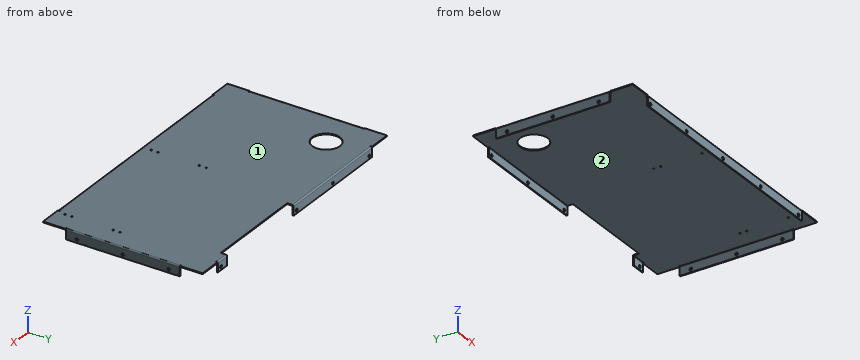
```python
from build123d import *

# Parameters (mm, degrees)
SM_BASE_FLANGE_1_DEPTH            = 2
SM_EDGE_FLANGE_1_STRIP_W          = 9.4732
SM_EDGE_FLANGE_1_STRIP_H          = 2
SM_EDGE_FLANGE_1_STRIP_CUT_DEPTH  = 248
SM_EDGE_FLANGE_1_RELIEF_W         = 10.4732
SM_EDGE_FLANGE_1_RELIEF_H         = 1
SM_EDGE_FLANGE_1_RELIEF_CUT_DEPTH = 2
SM_EDGE_FLANGE_1_DEPTH            = 248
SM_EDGE_FLANGE_2_STRIP_W          = 9.4732
SM_EDGE_FLANGE_2_STRIP_H          = 2
SM_EDGE_FLANGE_2_STRIP_CUT_DEPTH  = 510
SM_EDGE_FLANGE_2_RELIEF_W         = 10.4732
SM_EDGE_FLANGE_2_RELIEF_H         = 1
SM_EDGE_FLANGE_2_RELIEF_CUT_DEPTH = 2
SM_EDGE_FLANGE_2_DEPTH            = 510
SM_EDGE_FLANGE_3_STRIP_W          = 9.4732
SM_EDGE_FLANGE_3_STRIP_H          = 2
SM_EDGE_FLANGE_3_STRIP_CUT_DEPTH  = 248
SM_EDGE_FLANGE_3_RELIEF_W         = 10.4732
SM_EDGE_FLANGE_3_RELIEF_H         = 1
SM_EDGE_FLANGE_3_RELIEF_CUT_DEPTH = 2
SM_EDGE_FLANGE_3_DEPTH            = 248
SM_EDGE_FLANGE_4_STRIP_W          = 9.4732
SM_EDGE_FLANGE_4_STRIP_H          = 2
SM_EDGE_FLANGE_4_STRIP_CUT_DEPTH  = 31
SM_EDGE_FLANGE_4_RELIEF_W         = 10.4732
SM_EDGE_FLANGE_4_RELIEF_H         = 1
SM_EDGE_FLANGE_4_RELIEF_CUT_DEPTH = 2
SM_EDGE_FLANGE_4_DEPTH            = 31
SM_EDGE_FLANGE_5_STRIP_W          = 9.4732
SM_EDGE_FLANGE_5_STRIP_H          = 2
SM_EDGE_FLANGE_5_STRIP_CUT_DEPTH  = 259
SM_EDGE_FLANGE_5_RELIEF_W         = 10.4732
SM_EDGE_FLANGE_5_RELIEF_H         = 1
SM_EDGE_FLANGE_5_RELIEF_CUT_DEPTH = 2
SM_EDGE_FLANGE_5_DEPTH            = 259
HOLE_WIZARD_M4_1_D                = 3.3
HOLE_WIZARD_M4_1_DEPTH            = 10.1
HOLE_WIZARD_M4_1_TIP              = 0.991420021
SKETCH_20_R                       = 3
CUT_EXTRUDE_1_DEPTH               = 635.712533357
SKETCH_21_R                       = 3
CUT_EXTRUDE_2_DEPTH               = 464.263423983
SKETCH_22_R                       = 30
CUT_EXTRUDE_3_DEPTH               = 352.830925304


# Sheet-metal steps are written as plain solids
with BuildPart() as part:
    # Sketch 1 → 基体-法兰1 (new body)
    with BuildSketch(Plane.XY):
        Polygon((224, 174), (305, 174), (305, -174), (-305, -174), (-305, 174), (4, 174), (4, 160), (224, 160), align=None)
    extrude(amount=-SM_BASE_FLANGE_1_DEPTH)

    # 边线-法兰1 strip (across the edge) → 边线-法兰1 strip cut (cut)
    with BuildSketch(Plane(origin=(305, 124, -2), x_dir=(-1, 0, 0), z_dir=(0, -1, 0))):
        with Locations((-2, -1)):
            Rectangle(SM_EDGE_FLANGE_1_STRIP_W, SM_EDGE_FLANGE_1_STRIP_H)
    extrude(amount=SM_EDGE_FLANGE_1_STRIP_CUT_DEPTH, mode=Mode.SUBTRACT)

    # 边线-法兰1 relief (on the sheet) → 边线-法兰1 relief cut (cut)
    with BuildSketch(Plane(origin=(302.2634, 124, -2), x_dir=(-1, 0, 0), z_dir=(0, 0, -1))):
        with Locations((-4.2366, 0.5)):
            Rectangle(SM_EDGE_FLANGE_1_RELIEF_W, SM_EDGE_FLANGE_1_RELIEF_H)
        with Locations((-4.2366, -248.5)):
            Rectangle(SM_EDGE_FLANGE_1_RELIEF_W, SM_EDGE_FLANGE_1_RELIEF_H)
    extrude(amount=-SM_EDGE_FLANGE_1_RELIEF_CUT_DEPTH, mode=Mode.SUBTRACT)

    # 边线-法兰1 section (across the edge) → 边线-法兰1 (add)
    with BuildSketch(Plane(origin=(305, 124, -2), x_dir=(-1, 0, 0), z_dir=(0, -1, 0))):
        with BuildLine():
            Line((0, 0.7366), (0, 20))
            Line((0, 20), (2, 20))
            Line((2, 20), (2, 0.7366))
            ThreePointArc((2, 0.7366), (2.215745145, 0.215745145), (2.7366, 0))
            Line((2.7366, 0), (2.7366, -2))
            ThreePointArc((2.7366, -2), (0.801531583, -1.198468417), (0, 0.7366))
        make_face()
    extrude(amount=SM_EDGE_FLANGE_1_DEPTH)

    # 边线-法兰2 strip (across the edge) → 边线-法兰2 strip cut (cut)
    with BuildSketch(Plane(origin=(255, -174, -2), x_dir=(0, 1, 0), z_dir=(-1, 0, 0))):
        with Locations((-2, -1)):
            Rectangle(SM_EDGE_FLANGE_2_STRIP_W, SM_EDGE_FLANGE_2_STRIP_H)
    extrude(amount=SM_EDGE_FLANGE_2_STRIP_CUT_DEPTH, mode=Mode.SUBTRACT)

    # 边线-法兰2 relief (on the sheet) → 边线-法兰2 relief cut (cut)
    with BuildSketch(Plane(origin=(255, -171.2634, -2), x_dir=(0, 1, 0), z_dir=(0, 0, -1))):
        with Locations((-4.2366, 0.5)):
            Rectangle(SM_EDGE_FLANGE_2_RELIEF_W, SM_EDGE_FLANGE_2_RELIEF_H)
        with Locations((-4.2366, -510.5)):
            Rectangle(SM_EDGE_FLANGE_2_RELIEF_W, SM_EDGE_FLANGE_2_RELIEF_H)
    extrude(amount=-SM_EDGE_FLANGE_2_RELIEF_CUT_DEPTH, mode=Mode.SUBTRACT)

    # 边线-法兰2 section (across the edge) → 边线-法兰2 (add)
    with BuildSketch(Plane(origin=(255, -174, -2), x_dir=(0, 1, 0), z_dir=(-1, 0, 0))):
        with BuildLine():
            Line((0, 0.7366), (0, 20))
            Line((0, 20), (2, 20))
            Line((2, 20), (2, 0.7366))
            ThreePointArc((2, 0.7366), (2.215745145, 0.215745145), (2.7366, 0))
            Line((2.7366, 0), (2.7366, -2))
            ThreePointArc((2.7366, -2), (0.801531583, -1.198468417), (0, 0.7366))
        make_face()
    extrude(amount=SM_EDGE_FLANGE_2_DEPTH)

    # 边线-法兰3 strip (across the edge) → 边线-法兰3 strip cut (cut)
    with BuildSketch(Plane(origin=(-305, -124, -2), x_dir=(1, 0, 0), z_dir=(0, 1, 0))):
        with Locations((-2, -1)):
            Rectangle(SM_EDGE_FLANGE_3_STRIP_W, SM_EDGE_FLANGE_3_STRIP_H)
    extrude(amount=SM_EDGE_FLANGE_3_STRIP_CUT_DEPTH, mode=Mode.SUBTRACT)

    # 边线-法兰3 relief (on the sheet) → 边线-法兰3 relief cut (cut)
    with BuildSketch(Plane(origin=(-302.2634, -124, -2), x_dir=(1, 0, 0), z_dir=(0, 0, -1))):
        with Locations((-4.2366, 0.5)):
            Rectangle(SM_EDGE_FLANGE_3_RELIEF_W, SM_EDGE_FLANGE_3_RELIEF_H)
        with Locations((-4.2366, -248.5)):
            Rectangle(SM_EDGE_FLANGE_3_RELIEF_W, SM_EDGE_FLANGE_3_RELIEF_H)
    extrude(amount=-SM_EDGE_FLANGE_3_RELIEF_CUT_DEPTH, mode=Mode.SUBTRACT)

    # 边线-法兰3 section (across the edge) → 边线-法兰3 (add)
    with BuildSketch(Plane(origin=(-305, -124, -2), x_dir=(1, 0, 0), z_dir=(0, 1, 0))):
        with BuildLine():
            Line((0, 0.7366), (0, 20))
            Line((0, 20), (2, 20))
            Line((2, 20), (2, 0.7366))
            ThreePointArc((2, 0.7366), (2.215745145, 0.215745145), (2.7366, 0))
            Line((2.7366, 0), (2.7366, -2))
            ThreePointArc((2.7366, -2), (0.801531583, -1.198468417), (0, 0.7366))
        make_face()
    extrude(amount=SM_EDGE_FLANGE_3_DEPTH)

    # 边线-法兰4 strip (across the edge) → 边线-法兰4 strip cut (cut)
    with BuildSketch(Plane(origin=(224, 174, -2), x_dir=(0, -1, 0), z_dir=(1, 0, 0))):
        with Locations((-2, -1)):
            Rectangle(SM_EDGE_FLANGE_4_STRIP_W, SM_EDGE_FLANGE_4_STRIP_H)
    extrude(amount=SM_EDGE_FLANGE_4_STRIP_CUT_DEPTH, mode=Mode.SUBTRACT)

    # 边线-法兰4 relief (on the sheet) → 边线-法兰4 relief cut (cut)
    with BuildSketch(Plane(origin=(224, 171.2634, -2), x_dir=(0, -1, 0), z_dir=(0, 0, -1))):
        with Locations((-4.2366, -31.5)):
            Rectangle(SM_EDGE_FLANGE_4_RELIEF_W, SM_EDGE_FLANGE_4_RELIEF_H)
    extrude(amount=-SM_EDGE_FLANGE_4_RELIEF_CUT_DEPTH, mode=Mode.SUBTRACT)

    # 边线-法兰4 section (across the edge) → 边线-法兰4 (add)
    with BuildSketch(Plane(origin=(224, 174, -2), x_dir=(0, -1, 0), z_dir=(1, 0, 0))):
        with BuildLine():
            Line((0, 0.7366), (0, 20))
            Line((0, 20), (2, 20))
            Line((2, 20), (2, 0.7366))
            ThreePointArc((2, 0.7366), (2.215745145, 0.215745145), (2.7366, 0))
            Line((2.7366, 0), (2.7366, -2))
            ThreePointArc((2.7366, -2), (0.801531583, -1.198468417), (0, 0.7366))
        make_face()
    extrude(amount=SM_EDGE_FLANGE_4_DEPTH)

    # 边线-法兰5 strip (across the edge) → 边线-法兰5 strip cut (cut)
    with BuildSketch(Plane(origin=(-255, 174, -2), x_dir=(0, -1, 0), z_dir=(1, 0, 0))):
        with Locations((-2, -1)):
            Rectangle(SM_EDGE_FLANGE_5_STRIP_W, SM_EDGE_FLANGE_5_STRIP_H)
    extrude(amount=SM_EDGE_FLANGE_5_STRIP_CUT_DEPTH, mode=Mode.SUBTRACT)

    # 边线-法兰5 relief (on the sheet) → 边线-法兰5 relief cut (cut)
    with BuildSketch(Plane(origin=(-255, 171.2634, -2), x_dir=(0, -1, 0), z_dir=(0, 0, -1))):
        with Locations((-4.2366, 0.5)):
            Rectangle(SM_EDGE_FLANGE_5_RELIEF_W, SM_EDGE_FLANGE_5_RELIEF_H)
    extrude(amount=-SM_EDGE_FLANGE_5_RELIEF_CUT_DEPTH, mode=Mode.SUBTRACT)

    # 边线-法兰5 section (across the edge) → 边线-法兰5 (add)
    with BuildSketch(Plane(origin=(-255, 174, -2), x_dir=(0, -1, 0), z_dir=(1, 0, 0))):
        with BuildLine():
            Line((0, 0.7366), (0, 20))
            Line((0, 20), (2, 20))
            Line((2, 20), (2, 0.7366))
            ThreePointArc((2, 0.7366), (2.215745145, 0.215745145), (2.7366, 0))
            Line((2.7366, 0), (2.7366, -2))
            ThreePointArc((2.7366, -2), (0.801531583, -1.198468417), (0, 0.7366))
        make_face()
    extrude(amount=SM_EDGE_FLANGE_5_DEPTH)

    # M4 螺纹孔1
    with Locations(Plane.XY):
        with Locations((-24, -155), (-24, -140), (-24, -50), (-24, -35), (261, -155), (261, -140), (261, -50), (261, -35)):
            Hole(HOLE_WIZARD_M4_1_D / 2, depth=HOLE_WIZARD_M4_1_DEPTH)
            with Locations((0, 0, -(HOLE_WIZARD_M4_1_DEPTH + HOLE_WIZARD_M4_1_TIP / 2))):  # 118° drill point
                Cone(0, HOLE_WIZARD_M4_1_D / 2, HOLE_WIZARD_M4_1_TIP, mode=Mode.SUBTRACT)

    # 草图20 → 切除-拉伸1 (cut, through all)
    with BuildSketch(Plane(origin=(305, 0, 0), x_dir=(0, 0, -1), z_dir=(1, 0, 0))):
        with Locations((15, 0)):
            Circle(SKETCH_20_R)
        with Locations((15, 100)):
            Circle(SKETCH_20_R)
        with Locations((15, -100)):
            Circle(SKETCH_20_R)
    extrude(amount=-CUT_EXTRUDE_1_DEPTH, mode=Mode.SUBTRACT)

    # 草图21 → 切除-拉伸2 (cut, through all)
    with BuildSketch(Plane.XZ.offset(174)):
        with Locations(Location((-246, -15, 0), (0, 0, 270))):
            Circle(SKETCH_21_R)
        with Locations(Location((-126, -15, 0), (0, 0, 270))):
            Circle(SKETCH_21_R)
        with Locations(Location((-6, -15, 0), (0, 0, 270))):
            Circle(SKETCH_21_R)
        with Locations(Location((244, -15, 0), (0, 0, 270))):
            Circle(SKETCH_21_R)
        with Locations(Location((119, -15, 0), (0, 0, 270))):
            Circle(SKETCH_21_R)
    extrude(amount=-CUT_EXTRUDE_2_DEPTH, mode=Mode.SUBTRACT)

    # 草图22 → 切除-拉伸3 (cut, through all)
    with BuildSketch(Plane.XY):
        with Locations((-225, 94)):
            Circle(SKETCH_22_R)
    extrude(amount=-CUT_EXTRUDE_3_DEPTH, mode=Mode.SUBTRACT)


solid = part.part
```
Verification items for the finished model (mm, model axes). Face numbers are marked on the shaded views. Coordinates: 2 decimals unless noted, no trailing zeros. Order: outer loops, then holes, each group sorted by start corner. A loop starts at its lowest first (then second) coordinate and runs counter-clockwise, first axis right, second up. Notation, with made-up numbers: (5, 34.25) -> (62, 34.25) arc R19 ccw to (62, 49.25) -> close; hole circle Ø7 at (89, 75.25). An arc over 180 degrees is marked (long way). Answer as CSV lines item,"result". Start each with the question number.
1) Gauge pin test, flat ends, axial feed: pin 1 Ø1.9 at (y, z) = (172.5, -12) entering from -X; pin 2 Ø3 at (x, z) = (-303, -7.5) entering from +Y; pin 3 Ø4 at (x, y) = (-120, 77) entering from +Z; pin 4 Ø0.5 at (x, z) = (-255.5, -1) entering from +Y. Record the tip position at first contact, or that the pin passes through.
2) Cross-section at B-B, the plane x = 197. Record the boundary of the cut face in (y, z), then the cut area to 3 significant figures.
3) Material ranges on L1, parallel to Y at x = 304.55, z = -15; L2, parallel to Y at x = 261, z = -0.8; L3, parallel to X at y = -172.4, z = -15, recorded low to high. Write a range as [from, to].
4) Release check for a two-part mould opening along X. For the marked faces 1 and 2 record: released by +X, released by -X, zero draft, split by the parting line, or undercut.
5) Cross-section at A-A, the plane z = -7. Record the boundary of the cut face in (x, y), then the cut area to 3 significant figures.
6) Cross-section at D-D, the plane y = -132. Record the boundary of the cut face in (x, z), then the cut area to 3 significant figures.
7) Cross-section at C-C, the plane y = 77.5. Record the boundary of the cut face in (x, z).
Conclusion:
1,pin 1,"stops at x = -255"
1,pin 2,"stops at y = 124"
1,pin 3,"stops at z = 0"
1,pin 4,"stops at y = 170.26"
2,outline,"(-174, -22) -> (-172, -22) -> (-172, -2.74) arc R0.74 cw to (-171.26, -2) -> (160, -2) -> (160, 0) -> (-171.26, 0) arc R2.74 ccw to (-174, -2.74) -> close"
2,area,"707 mm²"
3,L1,"y = [-124, -103], [-97, -3], [3, 97], [103, 124]"
3,L2,"y = [-174, -156.65], [-153.35, -141.65], [-138.35, -51.65], [-48.35, -36.65], [-33.35, 174]"
3,L3,"x = [-255, -249], [-243, -129], [-123, -9], [-3, 116], [122, 241], [247, 255]"
4,face 1,"zero draft"
4,face 2,"undercut"
5,outline,"(-305, -124) -> (-303, -124) -> (-303, 124) -> (-305, 124) -> close; (-255, -174) -> (255, -174) -> (255, -172) -> (-255, -172) -> close; (-255, 172) -> (4, 172) -> (4, 174) -> (-255, 174) -> close; (224, 172) -> (255, 172) -> (255, 174) -> (224, 174) -> close; (303, -124) -> (305, -124) -> (305, 124) -> (303, 124) -> close"
5,area,"2,590 mm²"
6,outline,"(-305, -2) -> (305, -2) -> (305, 0) -> (-305, 0) -> close"
6,area,"1,220 mm²"
7,outline,"(-305, -22) -> (-303, -22) -> (-303, -2.74) arc R0.74 cw to (-302.26, -2) -> (-250.05, -2) -> (-250.05, 0) -> (-302.26, 0) arc R2.74 ccw to (-305, -2.74) -> close; (-199.95, -2) -> (302.26, -2) arc R0.74 cw to (303, -2.74) -> (303, -22) -> (305, -22) -> (305, -2.74) arc R2.74 ccw to (302.26, 0) -> (-199.95, 0) -> close"
